Verification items for this drawing (mm, ordinates from the low corner). Give positions to 0.01 mm unless a question says otherwise; leave off trailing zeros. Loops run counter-clockwise (first coordinate to the right, second up) from the corner with the lowest first, then second, coordinate; pieces in that order, holes last. Notation, with made-up numbers: (73.25, 21.25) -> (80.25, 21.25) arc R15 ccw to (80.25, 42.25) -> close; hole circle Ø7 at (66.5, 46.5). An arc over 180 degrees is marked (long way). Answer as CSV lines item,"result". Start each with the question number.
(1) Release check for a two-part mould opening along Z. For the marked faces 1, 2 and 3 record: pulls with the +Z half, pulls with the -Z half, needs draft (parallel to the pull), parting line crosses it, or undercut.
(2) Section check C-C on y = 68.5. Enter the section's corners in (x, z).
(3) Material ranges on line 1 (X direction, y = 39, z = 86); line 2 (X direction, y = 59, z = 120); line 3 (Z direction, x = 50, y = 53.5), recorded low to high. Write a range as from..to.
(4) Section check A-A on x = 550. Enter the section's corners in (y, z).
(5) Section check B-B on z = 107. Enter the section's corners in (x, y), plus the area to 3 significant figures.
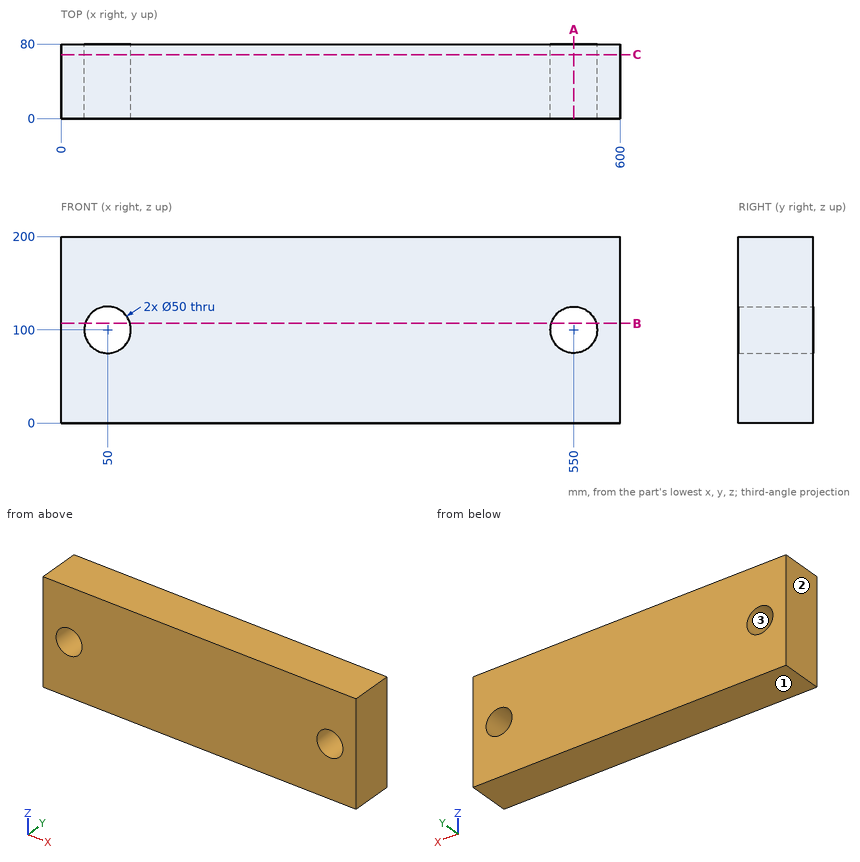
Working result:
1,face 1,"pulls with the -Z half"
1,face 2,"needs draft"
1,face 3,"undercut"
2,outline,"(0, 0) -> (600, 0) -> (600, 200) -> (0, 200) -> close; hole circle Ø50 at (50, 100); hole circle Ø50 at (550, 100)"
3,line 1,"x = 0..29.29, 70.71..529.29, 570.71..600"
3,line 2,"x = 0..35, 65..535, 565..600"
3,line 3,"z = 0..75, 125..200"
4,outline,"(0, 0) -> (80, 0) -> (80, 75) -> (0, 75) -> close; (0, 125) -> (80, 125) -> (80, 200) -> (0, 200) -> close"
5,outline,"(0, 0) -> (26, 0) -> (26, 80) -> (0, 80) -> close; (74, 0) -> (526, 0) -> (526, 80) -> (74, 80) -> close; (574, 0) -> (600, 0) -> (600, 80) -> (574, 80) -> close"
5,area,"40,300 mm^2"
